Answer from the drawing. Dimensions are ordinates in mm from the lowest x, y and z of the part. Give positions to 0.01 mm unless a question says otherwise; leave off trailing zeros. Loops run counter-clockwise (first coordinate to the right, second up) from the corner with the lowest first, then second, coordinate; pieces in that order, holes last.
(1) Find section C-C, the plane y = 13. Write down the section's boundary in (x, z).
(2) Each of these flat-tipped pins is pushed along its axis until it touches: P1, Ø1.5, axis at y = 18, z = 2, coming from the -X side; P2, Ø0.9, axis at x = 51.5, z = 2, coming from the -Y side; P3, Ø0.9, axis at x = 98, z = 1, coming from the +Y side. Where does it stop, or does it pass through?
(3) Straight lines are drawn through the part: probe 1 along Y at (x, z) = (60, 2.8); probe 2 along Y at (x, z) = (28, 2.5); probe 3 along X at (y, z) = (21.5, 0.15). For each, find the intervals that lie inside material, in ascending order.
(4) Find section B-B, the plane z = 0.6. State how many separate pieces and enclosed holes the cut face has, then the cut area to 3 significant figures.
(5) Find section A-A, the plane x = 79.5. Write down the section's boundary in (y, z), then the cut area to 3 significant figures.
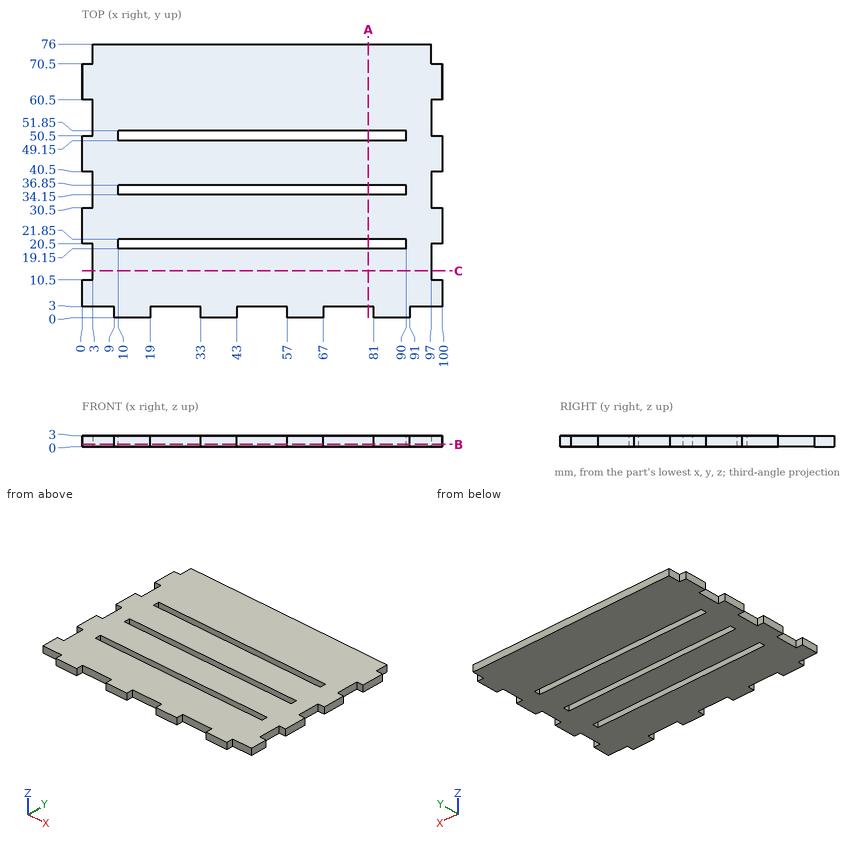
Entries:
1. outline: (3, 0) - (97, 0) - (97, 3) - (3, 3) - close
2. P1: stops at x = 3
2. P2: stops at y = 3
2. P3: stops at y = 70.5
3. probe 1: y = 0 to 19.15, 21.85 to 34.15, 36.85 to 49.15, 51.85 to 76
3. probe 2: y = 3 to 19.15, 21.85 to 34.15, 36.85 to 49.15, 51.85 to 76
3. probe 3: x = 0 to 10, 90 to 100
4. separate pieces: 1
4. enclosed holes: 3
4. area: 6,560 mm2
5. outline: (3, 0) - (19.15, 0) - (19.15, 3) - (3, 3) - close; (21.85, 0) - (34.15, 0) - (34.15, 3) - (21.85, 3) - close; (36.85, 0) - (49.15, 0) - (49.15, 3) - (36.85, 3) - close; (51.85, 0) - (76, 0) - (76, 3) - (51.85, 3) - close
5. area: 195 mm2
